from build123d import *

# Parameters (mm, degrees)
SKETCH1_W           = 100
SKETCH1_H           = 71
BOSS_EXTRUDE1_DEPTH = 3
FILLET4_R           = 3


with BuildPart() as part:
    # Sketch1 → Boss-Extrude1 (new body)
    with BuildSketch(Plane(origin=(0, 0, 0), x_dir=(1, 0, 0), z_dir=(0, 1, 0))):
        with Locations((-4.783432937, 2.318867117)):
            Rectangle(SKETCH1_W, SKETCH1_H)
    extrude(amount=BOSS_EXTRUDE1_DEPTH)

    # Fillet4
    fillet4_edges = [part.edges().sort_by_distance(p)[0] for p in [
        (-4.783432937, 3, -37.818867117),
        (45.216567063, 3, -2.318867117),
        (-4.783432937, 3, 33.181132883),
        (-54.783432937, 3, -2.318867117),
    ]]
    fillet(fillet4_edges, radius=FILLET4_R - 0.0001)  # a hair under: the kernel refuses the full size


solid = part.part
Verification items for the finished model (mm, model axes). Coordinates: 2 decimals unless noted, no trailing zeros. Write each loop counter-clockwise with the first axis right and the second up, starting at its lowest first coordinate (ties: lowest second). Pieces come first, ordered by that corner, then holes. Notation, with made-up numbers: (78, 37) -> (131, 37) arc R10 cw to (131, 41) -> close; hole circle Ø11 at (-5.5, -3). An arc over 180 degrees is marked (long way). One line per item, written item: value. Start each with the question number.
Q1. Go/stop test with a flat-tipped pin: P1, Ø1.5, axis at y = 1, z = -11.5, coming from the +X side. Record where the tip stops, or that it passes through.
Q2. Cross-section at B-B on y = 2.5. Enter the section's corners in (x, z).
Q3. Thickness scan on L1, parallel to Z at x = -22, y = 0.35; L2, parallel to X at y = 0.35, z = 19.5; L3, parallel to Z at x = -47.5, y = 1.7. Record the ranges inside material, lowest first. Write a range as from..to.
Checked values:
1. P1: stops at x = 45.21
2. outline: (-53.44, -36.48) -> (43.87, -36.48) -> (43.87, 31.84) -> (-53.44, 31.84) -> close
3. L1: z = -37.8..33.16
3. L2: x = -54.76..45.2
3. L3: z = -37.29..32.65
